from build123d import *

# Parameters (mm, degrees)
F0_W     = 160
F0_H     = 100
F1_DEPTH = 1.6
F3_D     = 3.3


with BuildPart() as f1:
    # F0 (on Top) → F1 (new body)
    with BuildSketch(Plane.XY):
        with Locations((80, 50)):
            Rectangle(F0_W, F0_H)
    extrude(amount=F1_DEPTH)

    # F3 (through all)
    with Locations(Plane.XY.offset(1.6)):
        with Locations((6.34, 93.18), (6.34, 6.82), (80, 6.82), (80, 93.18), (153.66, 93.18), (153.66, 6.82)):
            Hole(F3_D / 2)


solid = f1.part
For this review, take the finished solid that the model builds, in its own axes (mm). Give positions to 0.01 mm unless a question says otherwise; leave off trailing zeros. Loops run counter-clockwise (first coordinate to the right, second up) from the corner with the lowest first, then second, coordinate; pieces in that order, holes last. Notation, with made-up numbers: (0, -32.5) -> (33, -32.5) arc R17 cw to (33, -23.5) -> close; hole circle Ø9 at (1, 82.25). An arc over 180 degrees is marked (long way). One line per question, with ' | ' between items.
1) To check wall thickness, follow probe 1 along X at (y, z) = (93.18, 1.1); probe 2 along Y at (x, z) = (80, 1.25); probe 3 along X at (y, z) = (6, 0.8). State the ranges of each line that lie inside material, in increasing order.
Resolved:
probe 1: x = 0 to 4.69, 7.99 to 78.35, 81.65 to 152.01, 155.31 to 160 | probe 2: y = 0 to 5.17, 8.47 to 91.53, 94.83 to 100 | probe 3: x = 0 to 4.91, 7.77 to 78.57, 81.43 to 152.23, 155.09 to 160
2) Insertion check: pin 1 Ø2 at (x, y) = (6.34, 6.82) entering from -Z. The pin has a flat end and moves straight along its axis. Give the tip position at first contact, or say it passes through.
Resolved:
pin 1: passes through
3) The part is to be moulded in two halves that separate along Y. For faces 1 (the cylindrical face through (7.65, 5.82, 0.79)), 2 (the flat face through (79, 51, 0)), say which applies: +Y half, -Y half, draft (parallel to the pull), parting line (faces both ways), or undercut.
Resolved:
face 1: undercut | face 2: draft
4) We need section B-B (y = 93.18). Write out the cut boundary in (x, z).
Resolved:
outline: (0, 0) -> (4.69, 0) -> (4.69, 1.6) -> (0, 1.6) -> close; (7.99, 0) -> (78.35, 0) -> (78.35, 1.6) -> (7.99, 1.6) -> close; (81.65, 0) -> (152.01, 0) -> (152.01, 1.6) -> (81.65, 1.6) -> close; (155.31, 0) -> (160, 0) -> (160, 1.6) -> (155.31, 1.6) -> close
5) We need section A-A (x = 153.66). Write out the cut boundary in (y, z).
Resolved:
outline: (0, 0) -> (5.17, 0) -> (5.17, 1.6) -> (0, 1.6) -> close; (8.47, 0) -> (91.53, 0) -> (91.53, 1.6) -> (8.47, 1.6) -> close; (94.83, 0) -> (100, 0) -> (100, 1.6) -> (94.83, 1.6) -> close
